Autodesk Fusion 360 part; units mm, degrees
sketch "Base" plane through (0, 0, 0) normal (0, 0, 1) x (1, 0, 0) in component "Connector (AAA-Positive)"
  line L0 (4.7, -4.95) -> (-4.7, -4.95)
  line L1 (-4.7, -4.95) -> (-4.7, 4.95)
  line L2 (-4.7, 4.95) -> (4.7, 4.95)
  line L3 (4.7, 4.95) -> (4.7, -4.95)
  line L4 (4.7, -4.95) -> (-4.7, 4.95) construction
  line L5 (-4.7, -4.95) -> (4.7, 4.95) construction
  dimension "d1" = 9.4
  dimension "d2" = 9.9
extrude "Extrude1" add sketch "Base" along normal blind 0.4 in component "Connector (AAA-Positive)"
fillet "Fillet1" radius 0.5 4 edges at (4.7, -4.95, 0.2) (4.7, 4.95, 0.2) (-4.7, 4.95, 0.2) (-4.7, -4.95, 0.2) in component "Connector (AAA-Positive)"
sketch "Connector" plane through (4.7, 0, 0) normal (1, 0, 0) x (0, 1, 0) in component "Connector (AAA-Positive)"
  line L0 (4.45, 0) -> (4.45, 0.4)
  line L1 (4.45, 0.4) -> (-4.45, 0.4)
  line L2 (-4.45, 0.4) -> (-4.45, 0)
  line L3 (-4.45, 0) -> (4.45, 0)
  line L4 (-4.45, 0.2) -> (4.45, 0.2) construction
  line L5 (1.55, 0) -> (-1.55, 0)
  line L6 (-1.55, 0) -> (-1.55, 0.4)
  line L7 (-1.55, 0.4) -> (1.55, 0.4)
  line L8 (1.55, 0.4) -> (1.55, 0)
  line L9 (1.55, 0) -> (-1.55, 0.4) construction
  line L10 (-1.55, 0) -> (1.55, 0.4) construction
  point P0 (0, 0.2)
  dimension "d6" = 3.1
extrude "Extrude2" add sketch "Connector" along normal blind 6.7 contours L1 L3 L5 L6 L7 L8 in component "Connector (AAA-Positive)"
fillet "Fillet2" radius 1.55 2 edges at (11.4, -1.55, 0.2) (11.4, 1.55, 0.2) in component "Connector (AAA-Positive)"
sketch "Taps" plane through (0, 0, 0.4) normal (0, 0, 1) x (-1, 0, 0) in component "Connector (AAA-Positive)"
  arc A0 (-9.85, 1.55) -> (-9.85, -1.55) centre (-9.85, 0) ccw
  line L0 (-9.85, -1.55) -> (-4.7, -1.55)
  line L1 (-4.7, -1.55) -> (-4.7, -4.45)
  arc A1 (-4.7, -4.45) -> (-4.2, -4.95) centre (-4.2, -4.45) ccw
  line L2 (-4.2, -4.95) -> (4.2, -4.95)
  arc A2 (4.2, -4.95) -> (4.7, -4.45) centre (4.2, -4.45) ccw
  line L3 (4.7, -4.45) -> (4.7, 4.45)
  arc A3 (4.7, 4.45) -> (4.2, 4.95) centre (4.2, 4.45) ccw
  line L4 (4.2, 4.95) -> (-4.2, 4.95)
  arc A4 (-4.2, 4.95) -> (-4.7, 4.45) centre (-4.2, 4.45) ccw
  line L5 (-4.7, 4.45) -> (-4.7, 1.55)
  line L6 (-4.7, 1.55) -> (-9.85, 1.55)
  line L7 (4.7, 0) -> (-11.4, 0) construction
  line L8 (-9.85, -1.55) -> (-9.85, 1.55) construction
  circle A5 centre (-9.85, 0) radius 1
  line L9 (0, -4.95) -> (0, 4.95) construction
  circle A6 centre (0, 0) radius 2.5
  line L10 (-0.6, -3.05) -> (0.6, -3.05)
  line L11 (0.6, -3.05) -> (0.6, -4.55)
  line L12 (0.6, -4.55) -> (-0.6, -4.55)
  line L13 (-0.6, -4.55) -> (-0.6, -3.05)
  line L14 (-0.6, -3.05) -> (0.6, -4.55) construction
  line L15 (0.6, -3.05) -> (-0.6, -4.55) construction
  line L16 (-0.6, 4.55) -> (0.6, 4.55)
  line L17 (0.6, 4.55) -> (0.6, 3.05)
  line L18 (0.6, 3.05) -> (-0.6, 3.05)
  line L19 (-0.6, 3.05) -> (-0.6, 4.55)
  line L20 (-0.6, 4.55) -> (0.6, 3.05) construction
  line L21 (0.6, 4.55) -> (-0.6, 3.05) construction
  point P0 (0, -3.8)
  point P1 (0, 3.8)
  dimension "d10" = 1.55
  dimension "d11" = 2
  dimension "d12" = 5
  dimension "d13" = 1.2
  dimension "d14" = 1.5
  dimension "d15" = 0.4
  dimension "d16" = 1.2
  dimension "d17" = 1.5
  dimension "d18" = 0.4
extrude "Extrude3" cut sketch "Taps" against normal up to surface (0.4 mm away) contours A5 in component "Connector (AAA-Positive)"
extrude "Extrude4" add sketch "Taps" along normal blind 0.7 contours L10 L11 L12 L13 | L16 L17 L18 L19 in component "Connector (AAA-Positive)"
fillet "Fillet3" radius 0.5 4 edges at (0.6, 3.8, 1.1) (0.6, -3.8, 1.1) (-0.6, -3.8, 1.1) (-0.6, 3.8, 1.1) in component "Connector (AAA-Positive)"
extrude "Extrude5" add sketch "Taps" along normal blind 1.1 contours A6 in component "Connector (AAA-Positive)"
fillet "Fillet4" radius 1.1 1 edges at (2.3308, 0.904, 1.5) in component "Connector (AAA-Positive)"
component "Connector (AAA-Positive)" placed x (1, 0, 0) y (0, 1, 0) z (0, 0, 1) at (0, 0, 0)
The listing builds one solid part. Answer for the finished solid, in the listing's coordinates (mm). A direction names the side the tool comes from. Coordinates: 2 decimals unless noted, no trailing zeros. Write each loop counter-clockwise with the first axis right and the second up, starting at its lowest first coordinate (ties: lowest second). Pieces come first, ordered by that corner, then holes. Notation, with made-up numbers: (36, 71) - (93, 71) arc R18 cw to (93, 105) - close; hole circle Ø3 at (19.25, 5.5). An arc over 180 degrees is marked (long way). One line per item, written item: value.
1) Find section C-C (z = 0.9). Give the vertices of the cut face in (x, y), and give its area (3 significant figures).
Geometry check:
outline: circle Ø4.76 at (0, 0); (-0.5, -4.55) - (0.5, -4.55) - (0.5, -3.05) - (-0.5, -3.05) - close; (-0.5, 3.05) - (0.5, 3.05) - (0.5, 4.55) - (-0.5, 4.55) - close
area: 20.8 mm2
2) Consider line 1 along X through (y, z) = (0, 0.2); line 2 along Y through (x, z) = (9.85, 0.1); line 3 along Z through (x, y) = (-3, -3.25). Determine where each line is inside the solid, lowest interval first. Write a range as from..to.
Geometry check:
line 1: x = -4.7..8.85, 10.85..11.4
line 2: y = -1.55..-1, 1..1.55
line 3: z = 0..0.4
3) Find section D-D (x = 6.5). Give the vertices of the cut face in (y, z).
Geometry check:
outline: (-1.55, 0) - (1.55, 0) - (1.55, 0.4) - (-1.55, 0.4) - close
4) Each of these flat-tipped pins is pushed along its axis until it touches: pin 1 Ø2.5 at (x, y) = (9.85, 0) entering from +Z; pin 2 Ø0.8 at (x, z) = (0, 1) entering from +Y; pin 3 Ø0.6 at (x, z) = (0, 1) entering from -Y. Where does it stop, or does it pass through?
Geometry check:
pin 1: stops at z = 0.4
pin 2: stops at y = 4.55
pin 3: stops at y = -4.55
5) Find section A-A (x = 9.25). Give the vertices of the cut face in (y, z).
Geometry check:
outline: (-1.55, 0) - (-0.8, 0) - (-0.8, 0.4) - (-1.55, 0.4) - close; (0.8, 0) - (1.55, 0) - (1.55, 0.4) - (0.8, 0.4) - close
6) For a pull along X with two mould halves and no side action, classify faces 1 (the flat face through (0, 0, 1.5)), 2 (the cylindrical face through (10.85, -0.04, 0.2)), 3 (the cylindrical face through (10.93, -1.11, 0.2)) as pulls with the +X half, pulls with the -X half, needs draft (parallel to the pull), parting line crosses it, or undercut.
Geometry check:
face 1: needs draft
face 2: undercut
face 3: pulls with the +X half
7) A tool of negligible diameter and unlimited length cuts with its end or side. For faces 4 (the flat face through (3, 0, 0.4)), 5 (the cylindrical face through (10.93, 1.11, 0.2)), from which of +Z, -Z, +X, -X, +Y, -Y can it reach the whole face along a straight path? Write none if from no direction.
Geometry check:
face 4: +Z
face 5: +Z, -Z, +X, +Y
